Geometry: final body of the model. Coordinates: model frame, mm. A direction names the side the tool comes from. Round coordinates to 2 decimals unless told otherwise and drop trailing zeros. Loops run counter-clockwise (first coordinate to the right, second up) from the corner with the lowest first, then second, coordinate; pieces in that order, holes last. Notation, with made-up numbers: M -11.75,-38 L -4.75,-38 A25 cw -4.75,-1 Z; hole C 12,75 d10. An arc over 180 degrees is marked long. Answer as a JSON object with one key per item and string values.
from build123d import *

# Parameters (mm, degrees)
SKETCH1_W                                       = 330.2
SKETCH1_H                                       = 355.6
SKETCH1_R                                       = 76.2
BOSS_EXTRUDE1_DEPTH                             = 14.2875
CUT_EXTRUDE1_DEPTH                              = 2.2098
SKETCH2_R                                       = 76.2
CUT_EXTRUDE2_DEPTH                              = 3.175
SKETCH2_3_W                                     = 101.6
SKETCH2_3_H                                     = 42.8625
CUT_EXTRUDE3_DEPTH                              = 15.2875
FILLET1_R                                       = 6.604
FILLET2_R                                       = 6.35
FILLET3_R                                       = 1.27
F_1_4_20_TAPPED_HOLE1_D                         = 5.1054
F_10_24_TAPPED_HOLE1_D                          = 3.7973
CBORE_FOR_10_SOCKET_HEAD_CAP_SCREW2_D           = 5.1054
CBORE_FOR_10_SOCKET_HEAD_CAP_SCREW2_CBORE_D     = 8.636
CBORE_FOR_10_SOCKET_HEAD_CAP_SCREW2_CBORE_DEPTH = 4.826
F_10_24_TAPPED_HOLE2_D                          = 3.7973
F_10_24_TAPPED_HOLE2_DEPTH                      = 14.9606
F_10_24_TAPPED_HOLE2_TIP                        = 1.140824014
F_6_CLEARANCE_HOLE1_D                           = 3.7973


with BuildPart() as part:
    # Sketch1 → Boss-Extrude1 (new body)
    with BuildSketch(Plane.XY):
        with Locations((0, -14.2875)):
            Rectangle(SKETCH1_W, SKETCH1_H)
        Circle(SKETCH1_R, mode=Mode.SUBTRACT)
    extrude(amount=-BOSS_EXTRUDE1_DEPTH)

    # Sketch1_3 → Cut-Extrude1 (cut)
    with BuildSketch(Plane.XY):
        with BuildLine():
            Line((19.8628, -73.565679336), (19.8628, -192.0875))
            Line((19.8628, -192.0875), (61.1378, -192.0875))
            Line((61.1378, -192.0875), (61.1378, -45.481967978))
            ThreePointArc((61.1378, -45.481967978), (42.865464082, -62.999936421), (19.8628, -73.565679336))
        make_face()
    extrude(amount=-CUT_EXTRUDE1_DEPTH, mode=Mode.SUBTRACT)

    # Sketch2 → Cut-Extrude2 (cut)
    with BuildSketch(Plane(origin=(0, 0, -14.2875), x_dir=(-1, 0, 0), z_dir=(0, 0, -1))):
        with BuildLine():
            Line((50.8, 170.388379885), (50.8, 163.5125))
            Line((50.8, 163.5125), (-50.8, 163.5125))
            Line((-50.8, 163.5125), (-50.8, 170.388379885))
            ThreePointArc((-50.8, 170.388379885), (-111.466407665, 138.521045196), (-155.575, 86.077054869))
            Line((-155.575, 86.077054869), (-155.575, -86.077054869))
            ThreePointArc((-155.575, -86.077054869), (0, -177.8), (155.575, -86.077054869))
            Line((155.575, -86.077054869), (155.575, 86.077054869))
            ThreePointArc((155.575, 86.077054869), (111.466407665, 138.521045196), (50.8, 170.388379885))
        make_face()
        with Locations(Location((0, 0, 0), (0, 0, 216.646499469))):  # turned: the seam where the file's is
            Circle(SKETCH2_R, mode=Mode.SUBTRACT)
    extrude(amount=-CUT_EXTRUDE2_DEPTH, mode=Mode.SUBTRACT)

    # Sketch2_3 → Cut-Extrude3 (cut, through all)
    with BuildSketch(Plane(origin=(0, 0, -14.2875), x_dir=(-1, 0, 0), z_dir=(0, 0, -1))):
        with Locations((0, 142.08125)):
            Rectangle(SKETCH2_3_W, SKETCH2_3_H)
    extrude(amount=-CUT_EXTRUDE3_DEPTH, mode=Mode.SUBTRACT)

    # Fillet1
    fillet1_edges = [part.edges().sort_by_distance(p)[0] for p in [
        (-50.8, 163.5125, -5.55625),
        (50.8, 120.65, -5.55625),
        (-50.8, 120.65, -5.55625),
        (50.8, 163.5125, -5.55625),
    ]]
    fillet(fillet1_edges, radius=FILLET1_R)

    # Fillet2
    fillet2_edges = [part.edges().sort_by_distance(p)[0] for p in [
        (-155.575, 86.077054869, -12.7),
        (-155.575, -86.077054869, -12.7),
        (155.575, -86.077054869, -12.7),
        (155.575, 86.077054869, -12.7),
    ]]
    fillet(fillet2_edges, radius=FILLET2_R)

    # Fillet3
    fillet3_edges = [part.edges().sort_by_distance(p)[0] for p in [
        (69.831957897, 163.5125, -12.7),
        (-69.831957897, 163.5125, -12.7),
    ]]
    fillet(fillet3_edges, radius=FILLET3_R)

    # 1_4-20 Tapped Hole1 (through all)
    with Locations(Plane(origin=(0, 0, -11.1125), x_dir=(-1, 0, 0), z_dir=(0, 0, -1))):
        with Locations((-67.152219772, 150.826355057), (-138.464510768, 89.919904681), (-138.464510768, 0), (-138.464510768, -89.919904681), (-67.152219772, -150.826355057), (67.152219772, -150.826355057), (138.464510768, -89.919904681), (138.464510768, 0), (138.464510768, 89.919904681), (67.152219772, 150.826355057)):
            Hole(F_1_4_20_TAPPED_HOLE1_D / 2)

    # 10-24 Tapped Hole1 (through all)
    with Locations(Plane.XY.offset(-2.2098)):
        with Locations((54.7878, -83.1723), (54.7878, -168.8973), (38.9128, -143.4973)):
            Hole(F_10_24_TAPPED_HOLE1_D / 2)

    # CBORE for _10 Socket Head Cap Screw2 (through all)
    with Locations(Plane.XY):
        with Locations((-160.3375, -106.3625), (160.3375, -106.3625), (160.3375, -20.6375), (160.3375, 65.0875), (160.3375, 150.8125), (-160.3375, -20.6375), (-160.3375, 65.0875), (-160.3375, 150.8125)):
            CounterBoreHole(CBORE_FOR_10_SOCKET_HEAD_CAP_SCREW2_D / 2, CBORE_FOR_10_SOCKET_HEAD_CAP_SCREW2_CBORE_D / 2, CBORE_FOR_10_SOCKET_HEAD_CAP_SCREW2_CBORE_DEPTH)

    # 10-24 Tapped Hole2
    with Locations(Plane(origin=(0, -192.0875, 0), x_dir=(-1, 0, 0), z_dir=(0, -1, 0))):
        with Locations((76.2, 7.1501), (-76.2, 7.1501)):
            Hole(F_10_24_TAPPED_HOLE2_D / 2, depth=F_10_24_TAPPED_HOLE2_DEPTH)
            with Locations((0, 0, -(F_10_24_TAPPED_HOLE2_DEPTH + F_10_24_TAPPED_HOLE2_TIP / 2))):  # 118° drill point
                Cone(0, F_10_24_TAPPED_HOLE2_D / 2, F_10_24_TAPPED_HOLE2_TIP, mode=Mode.SUBTRACT)

    # 6 Clearance Hole1 (through all)
    with Locations(Plane.XY):
        with Locations((-160.3375, 106.2015)):
            Hole(F_6_CLEARANCE_HOLE1_D / 2)


solid = part.part
1) Pin query (flat end, axial travel): P1, Ø4, axis at x = 138.46, y = -89.92, coming from the +Z side; P2, Ø9.5, axis at x = 161.5, y = -106, coming from the +Z side; P3, Ø2.5, axis at x = -162, y = -20.5, coming from the +Z side. Return the tip coordinate at first contact, or that it passes through.
Results:
{"P1": "through", "P2": "z = 0", "P3": "z = -4.83"}
2) Section query D-D (x = 130). Return the cut outline in (y, z).
Results:
{"outline": "M -192.09,-14.29 L -121.3,-14.29 L -121.3,-11.11 L 121.3,-11.11 L 121.3,-14.29 L 163.51,-14.29 L 163.51,0 L -192.09,0 Z"}
3) Reachability of faces 1 (the flat face through (2, -81, -11.112)), 2 (the flat face through (-50, -172, -14.288)), 3 (the flat face through (-76, -12, 0)), 4 (the cylindrical face through (-164.65, 151, -2.38)), 5 (the flat face through (-50.8, 142, -6)) from +Z, -Z, +X, -X, +Y, -Y: full face, straight path, thin tool, end or side. Return the list, or none.
Results:
{"face 1": "-Z", "face 2": "-Z, +X, -X, +Y, -Y", "face 3": "+Z, +X, -X, +Y, -Y", "face 4": "+Z", "face 5": "+Z, -Z, +Y"}
4) Section query B-B (y = 17). Return the cut outline in (x, z) (1 decimal), and give its area (3 significant figures).
Results:
{"outline": "M -165.1,-14.3 L -155.6,-14.3 L -155.6,-11.1 L -74.3,-11.1 L -74.3,0 L -165.1,0 Z; M 74.3,-11.1 L 155.6,-11.1 L 155.6,-14.3 L 165.1,-14.3 L 165.1,0 L 74.3,0 Z", "area": "2,080 mm2"}
5) Ray query, line 1 (X direction, y = 4, z = -12.25) (3 decimals); line 2 (X direction, y = -22, z = -11.25) (3 decimals); line 3 (Y direction, x = 12.5, z = -10). Return the intervals inside material, ascending.
Results:
{"line 1": "-165.1 to -155.575, 155.575 to 165.1", "line 2": "-165.1 to -162.496, -158.179 to -155.575, 155.575 to 158.179, 162.496 to 165.1", "line 3": "-192.09 to -75.17, 75.17 to 120.65"}
6) Section query C-C (y = 99). Return the cut outline in (x, z), and give its area (3 significant figures).
Results:
{"outline": "M -165.1,-14.29 L -147.69,-14.29 L -147.69,-11.11 L 147.69,-11.11 L 147.69,-14.29 L 165.1,-14.29 L 165.1,0 L -165.1,0 Z", "area": "3,780 mm2"}
7) Pull-direction query (X, two-part tool) for faces 6 (the flat face through (40, -134, -2.21)), 7 (the flat face through (110, 163.513, -7)), 8 (the cylindrical face through (-164.65, -20.45, -2.38)); classes: +X half, -X half, draft (parallel to the pull), parting line (faces both ways), or undercut.
Results:
{"face 6": "undercut", "face 7": "draft", "face 8": "undercut"}
8) Section query A-A (x = 0). Return the cut outline in (y, z), and give its area (3 significant figures).
Results:
{"outline": "M -192.09,-14.29 L -177.8,-14.29 L -177.8,-11.11 L -76.2,-11.11 L -76.2,0 L -192.09,0 Z; M 76.2,-11.11 L 120.65,-11.11 L 120.65,0 L 76.2,0 Z", "area": "1,830 mm2"}
